The model under review builds one solid part; all positions refer to its coordinate system, in mm. A direction names the side the tool comes from. Round coordinates to 2 decimals unless told otherwise and drop trailing zeros. Loops run counter-clockwise (first coordinate to the right, second up) from the corner with the lowest first, then second, coordinate; pieces in that order, holes last. Notation, with made-up numbers: M 89.5,40 L 145.5,40 A12 ccw 145.5,45 Z; hole C 44,38 d10. An arc over 180 degrees is marked long. Answer as a JSON object with one key per item and string values. Group by question number.
Item 1: To check wall thickness, follow line 1 (Z direction, x = 0, y = 4); line 2 (Z direction, x = 0, y = 14.1); line 3 (Z direction, x = -9.5, y = 2.25). State the ranges of each line that lie inside material, in increasing order.
Item 2: Consider section B-B (y = 10.75). Give the boundary of the cut face in (x, z).
Item 3: Consider section A-A (y = 2.5). Give the boundary of the cut face in (x, z).
Item 4: Insertion check: P1, Ø10, axis at y = 10.5, z = -11, coming from the -X side; P2, Ø3, axis at x = 0, z = 9.5, coming from the -Y side; P3, Ø8, axis at y = 15, z = 7.5, coming from the -X side. Each pin has a flat end and moves straight along its axis. Give the tip position at first contact, or say it passes through.
Item 5: The part is to be moulded in two halves that separate along X. For faces 1 (the face through (-3, 15, 3)), 2 (the face through (0, 0, 0)), 3 (the face through (14.985, 8.902, -0.66)), say which applies: +X half, -X half, draft (parallel to the pull), parting line (faces both ways), or undercut.
Item 6: Tool access review of faces 4 (the face through (-6, 18, 0)), 5 (the face through (-0.07, 4.06, -7.88)), 6 (the face through (0, 13, 0)): name each direction out of +Z, -Z, +X, -X, +Y, -Y from which nothing blocks a thin tool from reaching the whole face with its end or side.
Autodesk Inventor part; units mm, degrees
ref_plane "YZ Plane" through (0, 0, 0) normal (1, 0, 0) x (0, 1, 0)
ref_plane "XZ Plane" through (0, 0, 0) normal (0, 1, 0) x (-1, 0, 0)
ref_plane "XY Plane" through (0, 0, 0) normal (0, 0, 1) x (1, 0, 0)
sketch "Sketch1" plane through (0, 0, 0) normal (0, 1, 0) x (-1, 0, 0)
  circle A0 centre (0, 0) radius 15
  dimension "d0" = 30
extrude "Extrusion1" add sketch "Sketch1" along normal blind 18
fillet "Fillet1" radius 2 2 edges at (15, 18, 0) (15, 0, 0)
sketch "Sketch4" plane through (0, 0, 0) normal (0, -1, 0) x (1, 0, 0)
  circle A0 centre (0, 0) radius 9.5 construction
  point P0 (0, 9.5)
  point P1 (0, -9.5)
  point P2 (-9.5, 0)
  point P3 (9.5, 0)
  dimension "d16" = 19
hole "Hole1" at (0, 0, 9.5) at (0, 0, -9.5) at (-9.5, 0, 0) at (9.5, 0, 0) direction (0, 1, 0) diameter 3.242 depth 8 tip angle 118
sketch "Sketch6" plane through (0, 18, 0) normal (0, 1, 0) x (1, 0, 0)
  line L0 (-3, 3) -> (3, 3) construction
  line L1 (3, 3) -> (3, -3) construction
  line L2 (3, -3) -> (-3, -3) construction
  line L3 (-3, -3) -> (-3, 3) construction
  circle A0 centre (0, 0) radius 4.2426
  dimension "d30" = 6
  dimension "d31" = 6
  dimension "d32" = 3
  dimension "d33" = 3
extrude "Extrusion6" cut sketch "Sketch6" against normal blind 5
chamfer "Chamfer1" distance 1 angle 60 1 edges at (-4.2426, 18, 0) measured on face at (-9.9139, 18, -1.3755)
properties part number "Motor"
Geometry results:
{
 "1": {"line 1": "z = -15 to -11.12, -7.88 to 7.88, 11.12 to 15", "line 2": "z = -15 to -4.24, 4.24 to 15", "line 3": "z = -11.61 to -1.62, 1.62 to 11.61"},
 "2": {"outline": "C 0,0 d30"},
 "3": {"outline": "C 0,0 d30; hole C -9.5,0 d3.24; hole C 0,-9.5 d3.24; hole C 0,9.5 d3.24; hole C 9.5,0 d3.24"},
 "4": {"P1": "stops at x = -13.75", "P2": "stops at y = 8.07", "P3": "stops at x = -14.59"},
 "5": {"face 1": "undercut", "face 2": "draft", "face 3": "parting line"},
 "6": {"face 4": "+Z, -Z, +X, -X, +Y", "face 5": "-Y", "face 6": "+Y"}
}
